For this review, take the finished solid that the model builds, in its own axes (mm). A direction names the side the tool comes from. Give positions to 0.01 mm unless a question says otherwise; leave off trailing zeros. Order: outer loops, then holes, each group sorted by start corner. A loop starts at its lowest first (then second) coordinate and runs counter-clockwise, first axis right, second up.
Item 1: Consider section A-A (x = -33). Give the boundary of the cut face in (y, z).
Item 2: For P1, Ø1.3, axis at y = 1, z = 1.5, coming from the +X side; P2, Ø1.5, axis at x = -9.5, y = 0.5, coming from the +Z side, all flat-tipped, find the tip position at first contact; note any pin that passes through.
Item 3: Machinability: for faces 1 (the flat face through (62.824, -2.467, 0.049)), 2 (the flat face through (6, 0, -2.3)), which of the approach directions +Z, -Z, +X, -X, +Y, -Y give a long, thin tool a straight path to every point of the face, cutting with its end or side? Answer none if there is none.
Item 4: Consider section B-B (z = -1). Give the boundary of the cut face in (x, y), plus the area to 3 significant figures.
Item 5: The part is to be moulded in two halves that separate along Y. For faces 3 (the flat face through (1, -2.25, 0)), 4 (the flat face through (-1, 0, -3.5)), 5 (the flat face through (-10, 3.5, 0)), say which applies: released by +Y, released by -Y, zero draft, split by the parting line, or undercut.
Item 6: For probe 1 along Z at (x, y) = (-61.5, -2); probe 2 along Y at (x, z) = (-38, -0.5); probe 3 along Y at (x, z) = (31, 2.5), list the stretches that pass through material, from the lowest coordinate up.
```python
from build123d import *

# Parameters (mm, degrees)
F0_W     = 150
F0_H     = 7
F1_DEPTH = 3.5
F2_W     = 1.7826502014
F2_H     = 1.2
F3_DEPTH = 140
F4_R     = 2
F6_DEPTH = 7.001


with BuildPart() as f1:
    # F0 (on Front) → F1 (new body, symmetric)
    with BuildSketch(Plane.XZ):
        Rectangle(F0_W, F0_H)
    extrude(amount=F1_DEPTH, both=True)

    # F2 (on face) → F3 (cut)
    with BuildSketch(Plane.YZ.offset(75)):
        with Locations((0, 2.9)):
            Rectangle(F2_W, F2_H)
        Polygon((-2.25, 2.3), (-2.25, -2.3), (2.25, -2.3), (2.25, 2.3), (0.8913251007, 2.3), (-0.8913251007, 2.3), align=None)
    extrude(amount=-F3_DEPTH, mode=Mode.SUBTRACT)

    # F4
    f4_edges = [f1.edges().sort_by_distance(p)[0] for p in [
        (-75, 3.5, 0),
        (-75, -3.5, 0),
    ]]
    fillet(f4_edges, radius=F4_R)

    # F5 (on face) → F6 (cut, through all)
    with BuildSketch(Plane.XY.offset(3.5)):
        Polygon((75, 3.5), (55, 3.5), (75, 0.8913251007), align=None)
        Polygon((75, -0.8913251007), (74.7628584504, -0.8913251007), (55, -3.5), (75, -3.5), align=None)
    extrude(amount=-F6_DEPTH, mode=Mode.SUBTRACT)


solid = f1.part
```
Resolved:
1. outline: (-3.5, -3.5) - (3.5, -3.5) - (3.5, 3.5) - (0.89, 3.5) - (0.89, 2.3) - (2.25, 2.3) - (2.25, -2.3) - (-2.25, -2.3) - (-2.25, 2.3) - (-0.89, 2.3) - (-0.89, 3.5) - (-3.5, 3.5) - close
2. P1: stops at x = -65
2. P2: stops at z = 3.5
3. face 1: +Z, -Z, +X, -Y
3. face 2: +X
4. outline: (-75, -1.5) arc R2 ccw to (-73, -3.5) - (55, -3.5) - (64.47, -2.25) - (-65, -2.25) - (-65, 2.25) - (64.58, 2.25) - (55, 3.5) - (-73, 3.5) arc R2 ccw to (-75, 1.5) - close
4. area: 380 mm2
5. face 3: undercut
5. face 4: zero draft
5. face 5: released by +Y
6. probe 1: z = -3.5 to -2.3, 2.3 to 3.5
6. probe 2: y = -3.5 to -2.25, 2.25 to 3.5
6. probe 3: y = -3.5 to -0.89, 0.89 to 3.5
